from build123d import *

# Parameters (mm, degrees)
F0_R     = 30
F0_R_2   = 27.5
F0_R_3   = 25
F1_DEPTH = 35
F2_DEPTH = 10
F3_R     = 27.5
F3_R_2   = 25
F4_DEPTH = 6


with BuildPart() as f1:
    # F0 (on Front) → F1 (new body)
    with BuildSketch(Plane.XZ):
        Circle(F0_R)
        Circle(F0_R_2, mode=Mode.SUBTRACT)
        Circle(F0_R_2)
        Circle(F0_R_3, mode=Mode.SUBTRACT)
    extrude(amount=F1_DEPTH)

    # F0 (on Front) → F2 (join)
    with BuildSketch(Plane.XZ):
        Circle(F0_R_2)
        Circle(F0_R_3, mode=Mode.SUBTRACT)
    extrude(amount=-F2_DEPTH)

    # F3 (on face) → F4 (join)
    with BuildSketch(Plane.XZ.offset(35)):
        Circle(F3_R)
        Circle(F3_R_2, mode=Mode.SUBTRACT)
    extrude(amount=F4_DEPTH)


solid = f1.part
Work out the finished part from the listing and answer in its coordinate system (mm). A direction names the side the tool comes from. Give positions to 0.01 mm unless a question says otherwise; leave off trailing zeros. Write each loop counter-clockwise with the first axis right and the second up, starting at its lowest first coordinate (ties: lowest second). Pieces come first, ordered by that corner, then holes. Notation, with made-up numbers: (-26.75, -20.5) - (12.25, -20.5) arc R21 ccw to (12.25, 17.5) - close; hole circle Ø9 at (10.25, 5.5). An arc over 180 degrees is marked (long way). One line per item, written item: value. Start each with the question number.
1. Consider probe 1 along Z at (x, y) = (0, -2.5); probe 2 along Z at (x, y) = (-14.5, -26.5); probe 3 along X at (y, z) = (-20.5, 6). Determine where each line is inside the solid, lowest interval first.
2. Given pin 1 (5 mm diameter, centred on x = 20, y = 3.5, fed in from -Z); pin 2 (6 mm diameter, centred on y = -10, z = 19, fed in from +X); pin 3 (2 mm diameter, centred on x = 18, y = -30.5, fed in from +Z), each flat-ended and moving along its own axis, determine where each tip first touches the part or whether it passes through.
3. For a pull along X with two mould halves and no side action, classify faces 4 (the cylindrical face through (23.846, -15.143, 7.509)), 5 (the flat face through (12.1, -41, -22.3)), 6 (the cylindrical face through (-5.961, 4.93, -26.846)) as +X half, -X half, draft (parallel to the pull), parting line (faces both ways), or undercut.
4. Find section C-C (y = -16). Write down the section's boundary in (x, z).
5. Find section B-B (x = 0). Write down the section's boundary in (y, z).
6. Find section A-A (z = 0). Write down the section's boundary in (x, y), then the cut area to 3 significant figures.
7. Find section D-D (y = 6). Write down the section's boundary in (x, z), then the cut area to 3 significant figures.
8. For faces 1 (the flat face through (12.1, 10, -22.3)), 2 (the flat face through (13.2, 0, -24.3)), 3 (the cylindrical face through (-5.961, -37.958, -26.846)), determine the directions among +Z, -Z, +X, -X, +Y, -Y from which every point of the face is accessible in a straight line to the end or side of a thin tool.
Geometry results:
1. probe 1: -30 to -25, 25 to 30
1. probe 2: -26.26 to -20.37, 20.37 to 26.26
1. probe 3: -29.39 to -24.27, 24.27 to 29.39
2. pin 1: z = -21.21
2. pin 2: x = 25.38
2. pin 3: z = 24.72
3. face 4: undercut
3. face 5: draft
3. face 6: parting line
4. outline: circle Ø60 at (0, 0); hole circle Ø50 at (0, 0)
5. outline: (-41, -27.5) - (-35, -27.5) - (-35, -30) - (0, -30) - (0, -27.5) - (10, -27.5) - (10, -25) - (-41, -25) - close; (-41, 25) - (10, 25) - (10, 27.5) - (0, 27.5) - (0, 30) - (-35, 30) - (-35, 27.5) - (-41, 27.5) - close
6. outline: (-30, -35) - (-27.5, -35) - (-27.5, -41) - (-25, -41) - (-25, 10) - (-27.5, 10) - (-27.5, 0) - (-30, 0) - close; (25, -41) - (27.5, -41) - (27.5, -35) - (30, -35) - (30, 0) - (27.5, 0) - (27.5, 10) - (25, 10) - close
6. area: 430 mm2
7. outline: circle Ø55 at (0, 0); hole circle Ø50 at (0, 0)
7. area: 412 mm2
8. face 1: +Z, -Z, +X, -X, +Y
8. face 2: +Y
8. face 3: -Y
